Check sheet for the modelled part. Datum: model origin and axes. Units: mm. A direction names the side the tool comes from. Coordinates: 2 decimals unless noted, no trailing zeros. Order: outer loops, then holes, each group sorted by start corner. A loop starts at its lowest first (then second) coordinate and runs counter-clockwise, first axis right, second up. Notation, with made-up numbers: M 9.25,23 L 58.25,23 A29 ccw 58.25,51 Z; hole C -38,66 d9. An arc over 180 degrees is marked long. Answer in a Markdown table with one row per item. Add a question column.
from build123d import *

# Parameters (mm, degrees)
BOSS_EXTRUDE1_START = 63.6
SKETCH1_R           = 9
BOSS_EXTRUDE1_DEPTH = 4
BOSS_EXTRUDE2_START = -100
SKETCH2_W           = 10
SKETCH2_H           = 4
BOSS_EXTRUDE2_DEPTH = 56.5
BOSS_EXTRUDE3_START = -104
SKETCH3_W           = 5
SKETCH3_H           = 26
BOSS_EXTRUDE3_DEPTH = 8
BOSS_EXTRUDE4_START = 63.1
SKETCH4_R           = 4.6
BOSS_EXTRUDE4_DEPTH = 2.3
BOSS_EXTRUDE5_START = -62
SKETCH5_W           = 6.6
SKETCH5_H           = 2.3
BOSS_EXTRUDE5_DEPTH = 17.5
BOSS_EXTRUDE6_START = -56.5
SKETCH6_W           = 1.8
SKETCH6_H           = 6
BOSS_EXTRUDE6_DEPTH = 10.5
BOSS_EXTRUDE7_START = -79.5
SKETCH7_W           = 6.6
SKETCH7_H           = 2.3
BOSS_EXTRUDE7_DEPTH = 17.5
BOSS_EXTRUDE8_START = -78
SKETCH8_W           = 1.8
SKETCH8_H           = 6
BOSS_EXTRUDE8_DEPTH = 10.5
BOSS_EXTRUDE9_START = 62.6
SKETCH9_R           = 3
BOSS_EXTRUDE9_DEPTH = 6


with BuildPart() as part:
    # Sketch1 → Boss-Extrude1 (new body)
    with BuildSketch(Plane(origin=(0, 0, 0), x_dir=(1, 0, 0), z_dir=(0, 1, 0)).offset(BOSS_EXTRUDE1_START)):
        with Locations(Location((0, 62, 0), (0, 0, 270))):
            Circle(SKETCH1_R)
    extrude(amount=BOSS_EXTRUDE1_DEPTH)

    # Sketch2 → Boss-Extrude2 (add)
    with BuildSketch(Plane.XY.offset(BOSS_EXTRUDE2_START)):
        with Locations((0, 65.6)):
            Rectangle(SKETCH2_W, SKETCH2_H)
    extrude(amount=BOSS_EXTRUDE2_DEPTH)

    # Sketch3 → Boss-Extrude3 (add)
    with BuildSketch(Plane.XY.offset(BOSS_EXTRUDE3_START)):
        with Locations((0, 76.6)):
            Rectangle(SKETCH3_W, SKETCH3_H)
    extrude(amount=BOSS_EXTRUDE3_DEPTH)


with BuildPart() as body_2:
    # Sketch4 → Boss-Extrude4 (new body)
    with BuildSketch(Plane(origin=(0, 0, 0), x_dir=(1, 0, 0), z_dir=(0, 1, 0)).offset(BOSS_EXTRUDE4_START)):
        with Locations(Location((0, 62, 0), (0, 0, 270))):
            Circle(SKETCH4_R)
    extrude(amount=BOSS_EXTRUDE4_DEPTH)


with BuildPart() as part_1:
    add(part.part)

    # Combine1: cut body 2
    add(body_2.part, mode=Mode.SUBTRACT)


with BuildPart() as body_2_2:
    # Sketch5 → Boss-Extrude5 (new body)
    with BuildSketch(Plane.XY.offset(BOSS_EXTRUDE5_START)):
        with Locations((0, 64.25)):
            Rectangle(SKETCH5_W, SKETCH5_H)
    extrude(amount=BOSS_EXTRUDE5_DEPTH)


with BuildPart() as part_2:
    add(part_1.part)

    # Combine2: cut body 2 2
    add(body_2_2.part, mode=Mode.SUBTRACT)


with BuildPart() as body_2_3:
    # Sketch6 → Boss-Extrude6 (new body)
    with BuildSketch(Plane.XY.offset(BOSS_EXTRUDE6_START)):
        with Locations((0, 65.6)):
            Rectangle(SKETCH6_W, SKETCH6_H)
    extrude(amount=BOSS_EXTRUDE6_DEPTH)


with BuildPart() as part_3:
    add(part_2.part)

    # Combine3: cut body 2 3
    add(body_2_3.part, mode=Mode.SUBTRACT)


with BuildPart() as body_2_4:
    # Sketch7 → Boss-Extrude7 (new body)
    with BuildSketch(Plane.XY.offset(BOSS_EXTRUDE7_START)):
        with Locations((0, 64.25)):
            Rectangle(SKETCH7_W, SKETCH7_H)
    extrude(amount=BOSS_EXTRUDE7_DEPTH)


with BuildPart() as part_4:
    add(part_3.part)

    # Combine4: cut body 2 4
    add(body_2_4.part, mode=Mode.SUBTRACT)


with BuildPart() as body_2_5:
    # Sketch8 → Boss-Extrude8 (new body)
    with BuildSketch(Plane.XY.offset(BOSS_EXTRUDE8_START)):
        with Locations((0, 65.6)):
            Rectangle(SKETCH8_W, SKETCH8_H)
    extrude(amount=BOSS_EXTRUDE8_DEPTH)


with BuildPart() as part_5:
    add(part_4.part)

    # Combine5: cut body 2 5
    add(body_2_5.part, mode=Mode.SUBTRACT)


with BuildPart() as body_2_6:
    # Sketch9 → Boss-Extrude9 (new body)
    with BuildSketch(Plane(origin=(0, 0, 0), x_dir=(1, 0, 0), z_dir=(0, 1, 0)).offset(BOSS_EXTRUDE9_START)):
        with Locations(Location((0, 62, 0), (0, 0, 270))):
            Circle(SKETCH9_R)
    extrude(amount=BOSS_EXTRUDE9_DEPTH)


with BuildPart() as part_6:
    add(part_5.part)

    # Combine6: cut body 2 6
    add(body_2_6.part, mode=Mode.SUBTRACT)


solid = part_6.part
1. Section check C-C on y = 71.25. Enter the section's corners in (x, z), then the cut area to 3 significant figures.
2. Section check D-D on x = 7.5. Enter the section's corners in (y, z).
3. Release check for a two-part mould opening along X. For faces 6 (the flat face through (-4, 66, -100)), 7 (the flat face through (-5, 66, -85)), 8 (the flat face through (-3.3, 64, -52)) record: released by +X, released by -X, zero draft, split by the parting line, or undercut.
4. Set-up check for faces 1 (the cylindrical face through (-9, 66, -62)), 2 (the flat face through (0, 67, -46)), 3 (the flat face through (3.3, 64, -72)), 4 (the flat face through (-5, 66, -49)), 5 (the cylindrical face through (9, 66, -62)): record each of +Z, -Z, +X, -X, +Y, -Y from which the full face is reachable in a straight line by a thin tool's end or side.
5. Go/stop test with flat-tipped pins: pin 1 Ø5.5 at (x, z) = (2.5, -84.5) entering from +Y; pin 2 Ø6.5 at (y, z) = (78.5, -98.5) entering from +X; pin 3 Ø6.5 at (y, z) = (82.5, -101.5) entering from -X. Record where each tip stops, or that it passes through.
6. Section check A-A on z = -73. Enter the section's corners in (x, y).
7. Scan lines: line 1 (Z direction, x = 0, y = 66.1); line 2 (Z direction, x = 3.25, y = 65); line 3 (Y direction, x = -2, z = -73). Record each from-to range of solid material in increasing order.
8. Section check B-B on z = -62. Enter the section's corners in (x, y).
Result sheet:
| question | item | result |
|---|---|---|
| 1 | outline | M -2.5,-104 L 2.5,-104 L 2.5,-96 L -2.5,-96 Z |
| 1 | area | 40.0 mm^2 |
| 2 | outline | M 63.6,-66.97 L 67.6,-66.97 L 67.6,-57.03 L 63.6,-57.03 Z |
| 3 | face 6 | zero draft |
| 3 | face 7 | released by -X |
| 3 | face 8 | undercut |
| 4 | face 1 | -X, +Y, -Y |
| 4 | face 2 | +Y, -Y |
| 4 | face 3 | -Y |
| 4 | face 4 | +Z, -X, +Y, -Y |
| 4 | face 5 | +X, +Y, -Y |
| 5 | pin 1 | y = 67.6 |
| 5 | pin 2 | x = 2.5 |
| 5 | pin 3 | x = -2.5 |
| 6 | outline | M -5,63.6 L -3.3,63.6 L -3.3,65.4 L -0.9,65.4 L -0.9,67.6 L -5,67.6 Z; M 0.9,65.4 L 3.3,65.4 L 3.3,63.6 L 5,63.6 L 5,67.6 L 0.9,67.6 Z |
| 7 | line 1 | -104 to -78, -67.5 to -65, -59 to -56.5, -46 to -43.5 |
| 7 | line 2 | -100 to -79.5, -44.5 to -43.5 |
| 7 | line 3 | 65.4 to 67.6 |
| 8 | outline | M -9,63.6 L -4.6,63.6 L -4.6,65.4 L -3,65.4 L -3,67.6 L -9,67.6 Z; M 3,65.4 L 4.6,65.4 L 4.6,63.6 L 9,63.6 L 9,67.6 L 3,67.6 Z |
